Autodesk Inventor part; units mm, degrees
ref_plane "YZ Plane" through (0, 0, 0) normal (1, 0, 0) x (0, 1, 0)
ref_plane "XZ Plane" through (0, 0, 0) normal (0, 1, 0) x (-1, 0, 0)
ref_plane "XY Plane" through (0, 0, 0) normal (0, 0, 1) x (1, 0, 0)
sketch "Sketch1" plane through (0, 0, 0) normal (1, 0, 0) x (0, 1, 0)
  line L0 (109, 0) -> (-109, 0) construction
  line L1 (147, 0) -> (-147, 0) construction
  line L2 (109, 0) -> (215.066, 0) construction
  line L3 (109, 0) -> (62.3692, 100)
  line L4 (109, 0) -> (219.3378, 0) construction
  line L5 (-147, 0) -> (3, 0) construction
  line L6 (-109, 0) -> (-62.3692, 100)
  line L7 (-109, 0) -> (1.3378, 0) construction
  line L8 (147, 0) -> (82.6495, 138)
  line L9 (82.6495, 138) -> (-82.6495, 138)
  line L10 (-82.6495, 138) -> (-147, 0)
  line L11 (62.3692, 100) -> (-62.3692, 100)
  line L12 (147, 0) -> (109, 0)
  line L13 (-109, 0) -> (-147, 0)
  line L14 (-62.3692, 100) -> (-82.6495, 138) construction
  line L15 (62.3338, 100) -> (82.6141, 138)
  line L16 (82.6661, 137.9646) -> (62.3858, 99.9646)
  line L17 (62.3692, 100) -> (82.6495, 138) construction
  line L18 (-62.3338, 100) -> (-82.6141, 138)
  line L19 (-82.6661, 137.9646) -> (-62.3858, 99.9646)
  point P0 (0, 0)
  point P1 (0, 0)
  point P2 (0, 0)
  dimension "d0" = 218
  dimension "d1" = 294
  dimension "d5" = 115
  dimension "d9" = 65
  dimension "d10" = 38
  dimension "d11" = 100
  dimension "d12" = 0.0625
  dimension "d13" = 0.0625
  dimension "d14" = 0.0312
  dimension "d15" = 0.0312
extrude "Extrusion1" add sketch "Sketch1" along normal blind 50 contours L3 L16 L8 L12 | L11 L18 L9 L15 | L6 L13 L10 L19
sketch "Sketch2" plane through (50, 0, 0) normal (1, 0, 0) x (0, 0, -1)
  line L0 (0, 109) -> (0, 147) construction
  line L1 (0, 147) -> (-137.9646, 82.6661) construction
  line L2 (-137.9646, 82.6661) -> (-99.9646, 62.3858) construction
  line L3 (-99.9646, 62.3858) -> (0, 109) construction
  line L4 (-100, 62.3338) -> (-138, 82.6141) construction
  line L5 (-138, 82.6141) -> (-138, -82.6141) construction
  line L6 (-138, -82.6141) -> (-100, -62.3338) construction
  line L7 (-100, -62.3338) -> (-100, 62.3338) construction
  line L8 (0, -109) -> (-99.9646, -62.3858) construction
  line L9 (-99.9646, -62.3858) -> (-137.9646, -82.6661) construction
  line L10 (-137.9646, -82.6661) -> (0, -147) construction
  line L11 (0, -147) -> (0, -109) construction
  line L12 (0, 109) -> (-100, 62.3692) construction
  line L13 (-100, 62.3692) -> (-100, -62.3692) construction
  line L14 (0, -109) -> (-99.9646, -62.3858) construction
  line L15 (-100, -62.3692) -> (0, -109) construction
  line L16 (0, -147) -> (0, -109) construction
  line L17 (0, -109) -> (0, -147) construction
  line L18 (0, -147) -> (-138, -82.6495) construction
  line L19 (-137.9646, -82.6661) -> (0, -147) construction
  line L20 (-138, -82.6495) -> (-138, 82.6495) construction
  line L21 (0, 109) -> (0, 147) construction
  line L22 (-138, 82.6495) -> (0, 147) construction
  line L23 (0, 147) -> (0, 109) construction
  line L24 (-106.5, 66.5102) -> (0, 116.172)
  line L25 (0, 139.828) -> (-131.5, 78.5086)
  line L26 (-131.5, 78.5086) -> (-131.5, -78.5086)
  line L27 (-131.5, -78.5086) -> (0, -139.828)
  line L28 (0, -116.172) -> (-106.5, -66.5102)
  line L29 (-106.5, -66.5102) -> (-106.5, 66.5102)
  line L30 (0, -147) -> (0, -109)
  line L31 (0, 139.828) -> (0, 116.172)
  line L32 (0, -116.172) -> (0, -139.828)
  point P0 (0, 0)
  dimension "d18" = 6.5
extrude "Extrusion2" cut sketch "Sketch2" against normal blind 43.5
extrude "Extrusion3" add sketch "Sketch2" against normal blind 6.5
properties part number "FrameMainMotorMount"
Read the model definition and answer for the solid it produces. Units are mm, in the model's axes. A direction names the side the tool comes from. Give positions to 0.01 mm unless a question says otherwise; leave off trailing zeros. Loops run counter-clockwise (first coordinate to the right, second up) from the corner with the lowest first, then second, coordinate; pieces in that order, holes last. Notation, with made-up numbers: (78, -15) -> (137, -15) arc R17 cw to (137, 2) -> close; hole circle Ø4 at (2.25, 80). An arc over 180 degrees is marked (long way). Use a Markdown table: item, result.
Q1. Determine the mould class of faces 1 (the face through (0, -1, 119)), 2 (the face through (6.5, 98, 61)), 3 (the face through (25, 1, 138)) for opening direction X: pulls with the +X half, pulls with the -X half, needs draft (parallel to the pull), parting line crosses it, or undercut.
Solved:
| item | result |
|---|---|
| face 1 | pulls with the -X half |
| face 2 | undercut |
| face 3 | needs draft |
Q2. Section A-A, the plane y = 1 is taken. Determine the outline of the cut face in (x, z), then the cut area to 3 significant figures.
Solved:
| item | result |
|---|---|
| outline | (0, 100) -> (50, 100) -> (50, 138) -> (0, 138) -> close; hole (6.5, 106.5) -> (43.5, 106.5) -> (43.5, 131.5) -> (6.5, 131.5) -> close |
| area | 975 mm^2 |
Q3. A tool of negligible diameter and unlimited length cuts with its end or side. For faces 4 (the face through (25, 1, 100)), 5 (the face through (50, 2, 101)), 6 (the face through (25.26, -91.69, 52.5)), from which of +Z, -Z, +X, -X, +Y, -Y can it reach the whole face along a straight path? Write none if from no direction.
Solved:
| item | result |
|---|---|
| face 4 | -Z, +X, -X |
| face 5 | +Z, -Z, +X, +Y, -Y |
| face 6 | none |
Q4. Section C-C, the plane x = 15 is taken. Determine the outline of the cut face in (y, z).
Solved:
| item | result |
|---|---|
| outline | (-147, 0) -> (-139.83, 0) -> (-78.84, 130.79) -> (-82.67, 137.96) -> close; (-116.17, 0) -> (-109, 0) -> (-62.39, 99.96) -> (-65.87, 106.5) -> (-66.51, 106.5) -> close; (-82.61, 138) -> (-78.81, 130.86) -> (-78.51, 131.5) -> (78.51, 131.5) -> (78.81, 130.86) -> (82.61, 138) -> close; (-65.8, 106.5) -> (-62.33, 100) -> (62.33, 100) -> (65.8, 106.5) -> close; (62.39, 99.96) -> (109, 0) -> (116.17, 0) -> (66.51, 106.5) -> (65.87, 106.5) -> close; (78.84, 130.79) -> (139.83, 0) -> (147, 0) -> (82.67, 137.96) -> close |
Q5. Section B-B, the plane z = 23 is taken. Determine the outline of the cut face in (x, y), then the cut area to 3 significant figures.
Solved:
| item | result |
|---|---|
| outline | (0, -136.27) -> (50, -136.27) -> (50, -98.27) -> (0, -98.27) -> close; (0, 98.27) -> (50, 98.27) -> (50, 136.27) -> (0, 136.27) -> close; hole (6.5, -129.1) -> (43.5, -129.1) -> (43.5, -105.45) -> (6.5, -105.45) -> close; hole (6.5, 105.45) -> (43.5, 105.45) -> (43.5, 129.1) -> (6.5, 129.1) -> close |
| area | 2,050 mm^2 |
Q6. Section D-D, the plane z = 115.5 is taken. Determine the outline of the cut face in (x, y).
Solved:
| item | result |
|---|---|
| outline | (0, -93.14) -> (50, -93.14) -> (50, 93.14) -> (0, 93.14) -> (0, 70.68) -> (6.5, 70.68) -> (6.5, 85.97) -> (43.5, 85.97) -> (43.5, -85.97) -> (6.5, -85.97) -> (6.5, -70.68) -> (0, -70.68) -> close; (0, -70.61) -> (6.5, -70.61) -> (6.5, 70.61) -> (0, 70.61) -> close |
Q7. Find the intervals of material crossed by line 1 along X through (y, z) = (45, 126); line 2 along Y through (x, z) = (33.5, 40); line 3 along Y through (x, z) = (33.5, 97.5), in increasing order.
Solved:
| item | result |
|---|---|
| line 1 | x = 0 to 6.5, 43.5 to 50 |
| line 2 | y = -128.35 to -121.18, -97.52 to -90.35, 90.35 to 97.52, 121.18 to 128.35 |
| line 3 | y = -101.53 to -94.36, -70.71 to -63.53, 63.53 to 70.71, 94.36 to 101.53 |
Q8. Each of these flat-tipped pins is pushed along its axis until it touches: pin 1 (2 mm diameter, centred on x = 11.5, y = 63.5, fed in from -Z); pin 2 (12 mm diameter, centred on x = 24.5, z = 24.5, fed in from +Y); pin 3 (1.5 mm diameter, centred on x = 20, y = 63, fed in from -Z). Where does it stop, or does it pass through?
Solved:
| item | result |
|---|---|
| pin 1 | stops at z = 95.43 |
| pin 2 | stops at y = 138.37 |
| pin 3 | stops at z = 97.04 |
